from build123d import *

# Parameters (mm, degrees)
BOSS_EXTRUDE1_DEPTH = 3
SKETCH2_W           = 7
SKETCH2_H           = 3
CUT_EXTRUDE1_DEPTH  = 10


with BuildPart() as part:
    # Sketch1 → Boss-Extrude1 (new body)
    with BuildSketch(Plane(origin=(0, 0, 0), x_dir=(0, 0, -1), z_dir=(1, 0, 0))):
        Polygon((0, 20), (-15, 0), (-12, 0), (-12, -3), (-7, -3), (-7, 0), (0, 0), (0, 3), (3, 3), (3, 8), (0, 8), align=None)
    extrude(amount=BOSS_EXTRUDE1_DEPTH)

    # Sketch2 → Cut-Extrude1 (cut)
    with BuildSketch(Plane(origin=(3, 0, 0), x_dir=(0, 0, -1), z_dir=(1, 0, 0))):
        with Locations((-3.5, 1.5)):
            Rectangle(SKETCH2_W, SKETCH2_H)
    extrude(amount=-CUT_EXTRUDE1_DEPTH, mode=Mode.SUBTRACT)


solid = part.part
Can you work these out from the model? Positions are in its coordinate system, mm. A direction names the side the tool comes from. Give positions to 0.01 mm unless a question says otherwise; leave off trailing zeros. Loops run counter-clockwise (first coordinate to the right, second up) from the corner with the lowest first, then second, coordinate; pieces in that order, holes last. Notation, with made-up numbers: (-29.5, 7) -> (-3.5, 7) arc R9 cw to (-3.5, 19) -> close; hole circle Ø11 at (-13.5, 4). An arc over 180 degrees is marked (long way). Return JSON: item names as keys, results as strings.
Q1. I want a section at B-B, the plane y = -1. List the corners of the cut face in (x, z) for me, then the cut area to 3 significant figures.
Checks:
{"outline": "(0, 7) -> (3, 7) -> (3, 12) -> (0, 12) -> close", "area": "15.0 mm2"}
Q2. I need wall thicknesses on probe 1 along Y at (x, z) = (1.05, 6); probe 2 along Z at (x, y) = (1.45, -2); probe 3 along Y at (x, z) = (0.75, -0.75). Which ranges of each line are inside material? Lowest first, please.
Checks:
{"probe 1": "y = 3 to 12", "probe 2": "z = 7 to 12", "probe 3": "y = 3 to 8"}
Q3. I want a section at A-A, the plane x = 1.3. List the corners of the cut face in (y, z) for me.
Checks:
{"outline": "(-3, 7) -> (3, 7) -> (3, -3) -> (8, -3) -> (8, 0) -> (20, 0) -> (0, 15) -> (0, 12) -> (-3, 12) -> close"}
Q4. For pin 1 Ø1.5 at (x, z) = (2, 2) entering from -Y; pin 2 Ø1.5 at (x, y) = (1, -2) entering from +Z; pin 3 Ø1.5 at (x, y) = (2, 15.5) entering from -Z, each with a flat end and sliding along its axis, tell me the tip position at first contact or that it passes through.
Checks:
{"pin 1": "stops at y = 3", "pin 2": "stops at z = 12", "pin 3": "stops at z = 0"}
Q5. On a 3-axis mill with a long thin cutter (end or side, diameter ignored), from which of +Z, -Z, +X, -X, +Y, -Y can I reach the whole of each face in a straight line? I mean faces 1 (the face through (1, 8, -2)), 2 (the face through (1, -1, 12)), 3 (the face through (2, 0, 7)). Say none if no direction works.
Checks:
{"face 1": "-Z, +X, -X, +Y", "face 2": "+Z, +X, -X, -Y", "face 3": "-Z, +X, -X, -Y"}
Q6. I want a section at C-C, the plane z = 8.25. List the corners of the cut face in (x, y) for me, then the cut area to 3 significant figures.
Checks:
{"outline": "(0, -3) -> (3, -3) -> (3, 9) -> (0, 9) -> close", "area": "36.0 mm2"}
